from build123d import *

# Parameters (mm, degrees)
F0_R     = 22.225
F1_DEPTH = 50.8
F2_T     = -6.35
F3_R     = 0.635


with BuildPart() as f1:
    # F0 (on Top) → F1 (new body)
    with BuildSketch(Plane.XY):
        Circle(F0_R)
    extrude(amount=F1_DEPTH)

    # F2
    f2_openings = [f1.faces().sort_by_distance(p)[0] for p in [
        (0, 0, 50.8),
        (0, 0, 0),
    ]]
    offset(amount=F2_T, openings=f2_openings)

    # F3
    f3_edges = [f1.edges().sort_by_distance(p)[0] for p in [
        (-22.225, 0, 50.8),
        (-15.875, 0, 50.8),
    ]]
    fillet(f3_edges, radius=F3_R)


solid = f1.part
Work out the finished part from the listing and answer in its coordinate system (mm). Coordinates: 2 decimals unless noted, no trailing zeros. Write each loop counter-clockwise with the first axis right and the second up, starting at its lowest first coordinate (ties: lowest second). Pieces come first, ordered by that corner, then holes.
1. The part is cut by section A-A, the plane x = 0. Write down the section's boundary in (y, z) (3 decimals).
Results list:
outline: (-22.225, 0) - (-15.875, 0) - (-15.875, 50.165) arc R0.635 ccw to (-16.51, 50.8) - (-21.59, 50.8) arc R0.635 ccw to (-22.225, 50.165) - close; (15.875, 0) - (22.225, 0) - (22.225, 50.165) arc R0.635 ccw to (21.59, 50.8) - (16.51, 50.8) arc R0.635 ccw to (15.875, 50.165) - close
2. Consider line 1 along Y through (x, z) = (0, 28.5) (3 decimals); line 2 along X through (y, z) = (1, 20.5); line 3 along X through (y, z) = (8, 20). Determine where each line is inside the solid, lowest interval first.
Results list:
line 1: y = -22.225 to -15.875, 15.875 to 22.225
line 2: x = -22.2 to -15.84, 15.84 to 22.2
line 3: x = -20.74 to -13.71, 13.71 to 20.74
3. For a pull along Y with two mould halves and no side action, classify faces 1 (the cylindrical face through (21.199, 6.676, 24.731)), 2 (the cylindrical face through (-3.441, -15.497, 24.731)), 3 (the flat face through (-5, -16, 50.8)) as +Y half, -Y half, draft (parallel to the pull), parting line (faces both ways), or undercut.
Results list:
face 1: parting line
face 2: undercut
face 3: draft
4. The part is cut by section C-C, the plane z = 39.5. Write down the section's boundary in (x, y) (3 decimals), and give its area (3 significant figures).
Results list:
outline: circle Ø44.45 at (0, 0); hole circle Ø31.75 at (0, 0)
area: 760 mm2
5. Flat-ended cylindrical pins translate along their axes: pin 1 (5 mm diameter, centred on y = 3.5, z = 15.5, fed in from +X); pin 2 (8 mm diameter, centred on y = 15.5, z = 23.5, fed in from -X); pin 3 (10 mm diameter, centred on x = 10.5, z = 43, fed in from -Y). Find the tip coordinate at first contact, or state that the pin passes through.
Results list:
pin 1: stops at x = 22.2
pin 2: stops at x = -19.02
pin 3: stops at y = -21.53
